Drawing for the job (mm, zero at the part's lowest x, y, z). Round coordinates to 2 decimals unless told otherwise and drop trailing zeros. Write each loop counter-clockwise with the first axis right and the second up, starting at its lowest first coordinate (ties: lowest second). Pieces come first, ordered by that corner, then holes. Notation, with made-up numbers: (76.5, -11) -> (80.5, -11) arc R11 ccw to (80.5, -1) -> close; hole circle Ø3 at (19.25, -16). An arc over 180 degrees is marked (long way). Answer in a Markdown table with one row per item. Add a question column.
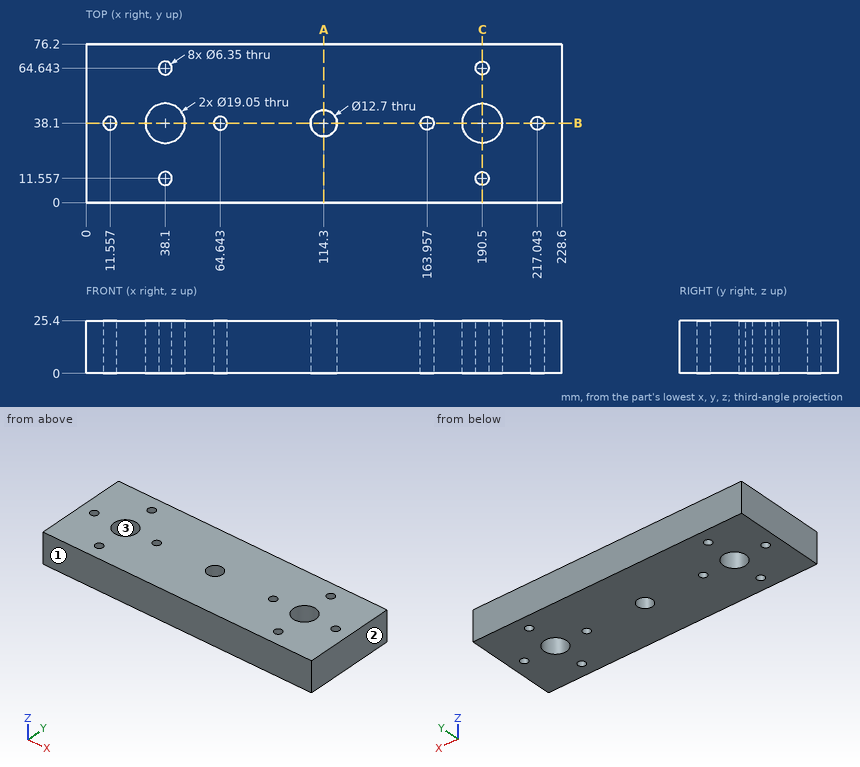
(1) Probe line 1 along Y through (x, z) = (38.1, 7.25) (3 decimals); line 2 along Y through (x, z) = (189.5, 19); line 3 along X through (y, z) = (45, 3.5). List the from-to ranges inside material, lowest first.
(2) Drop a flat-ended pin along its axis: P1, Ø8.5, axis at x = 38.1, y = 11.557, coming from the -Z side. Give the stop position or say it passes through.
(3) Saw through at B-B (y = 38.1). Count the separate pieces of the cut face and the enclosed holes in it, plus the area to 3 significant figures.
(4) Mould opens along Y. For the marked faces 1, 2 and 3 say: pulls with the +Y half, pulls with the -Y half, needs draft (parallel to the pull), parting line crosses it, or undercut.
(5) Saw through at C-C (x = 190.5). List the corners of the cut face in (y, z) (3 decimals).
(6) Saw through at A-A (x = 114.3). List the corners of the cut face in (y, z).
Answer sheet:
| question | item | result |
|---|---|---|
| 1 | line 1 | y = 0 to 8.382, 14.732 to 28.575, 47.625 to 61.468, 67.818 to 76.2 |
| 1 | line 2 | y = 0 to 8.54, 14.57 to 28.63, 47.57 to 61.63, 67.66 to 76.2 |
| 1 | line 3 | x = 0 to 31.53, 44.67 to 183.93, 197.07 to 228.6 |
| 2 | P1 | stops at z = 0 |
| 3 | separate pieces | 8 |
| 3 | enclosed holes | 0 |
| 3 | area | 3,870 mm² |
| 4 | face 1 | pulls with the -Y half |
| 4 | face 2 | needs draft |
| 4 | face 3 | undercut |
| 5 | outline | (0, 0) -> (8.382, 0) -> (8.382, 25.4) -> (0, 25.4) -> close; (14.732, 0) -> (28.575, 0) -> (28.575, 25.4) -> (14.732, 25.4) -> close; (47.625, 0) -> (61.468, 0) -> (61.468, 25.4) -> (47.625, 25.4) -> close; (67.818, 0) -> (76.2, 0) -> (76.2, 25.4) -> (67.818, 25.4) -> close |
| 6 | outline | (0, 0) -> (31.75, 0) -> (31.75, 25.4) -> (0, 25.4) -> close; (44.45, 0) -> (76.2, 0) -> (76.2, 25.4) -> (44.45, 25.4) -> close |
